```python
from build123d import *

# Parameters (mm, degrees)
SALIENTE_EXTRUIR1_DEPTH = 30
CORTAR_EXTRUIR1_DEPTH   = 5
CROQUIS3_W              = 30
CROQUIS3_H              = 25
CORTAR_EXTRUIR2_DEPTH   = 2
CROQUIS4_R              = 1.35
CROQUIS4_R_2            = 3
CORTAR_EXTRUIR3_DEPTH   = 5
CROQUIS5_W              = 25
CROQUIS5_H              = 25
CORTAR_EXTRUIR4_DEPTH   = 2
REDONDEO1_R             = 15
REDONDEO2_R             = 8
REDONDEO3_R             = 2.7
SALIENTE_EXTRUIR2_DEPTH = 5
REDONDEO4_R             = 5
SALIENTE_EXTRUIR3_START = -3
SALIENTE_EXTRUIR3_DEPTH = 3
SALIENTE_EXTRUIR4_START = -30
SALIENTE_EXTRUIR4_DEPTH = 3
REDONDEO5_R             = 10


with BuildPart() as part:
    # Croquis1 → Saliente-Extruir1 (new body)
    with BuildSketch(Plane.XY):
        with BuildLine():
            Line((0, 0), (0, 5))
            Line((0, 5), (-40, 5))
            ThreePointArc((-40, 5), (-59.427874629, -2.62943546), (-71, -20))
            Line((-71, -20), (-71, -60))
            Line((-71, -60), (-66, -60))
            Line((-66, -60), (-66, -20.535714286))
            ThreePointArc((-66, -20.535714286), (-56.328368106, -6.472823549), (-40.535714286, 0))
            Line((-40.535714286, 0), (0, 0))
        make_face()
    extrude(amount=SALIENTE_EXTRUIR1_DEPTH)

    # Croquis2 → Cortar-Extruir1 (cut)
    with BuildSketch(Plane(origin=(0, 5, 0), x_dir=(1, 0, 0), z_dir=(0, 1, 0))):
        with BuildLine():
            Line((-18.4, -6.93), (-8.4, -6.93))
            ThreePointArc((-8.4, -6.93), (-7.05, -8.28), (-8.4, -9.63))
            Line((-8.4, -9.63), (-28.4, -9.63))
            ThreePointArc((-28.4, -9.63), (-29.75, -8.28), (-28.4, -6.93))
            Line((-28.4, -6.93), (-18.4, -6.93))
        make_face()
        with BuildLine():
            Line((-8.4, -20.37), (-28.4, -20.37))
            ThreePointArc((-28.4, -20.37), (-29.75, -21.72), (-28.4, -23.07))
            Line((-28.4, -23.07), (-18.4, -23.07))
            Line((-18.4, -23.07), (-8.4, -23.07))
            ThreePointArc((-8.4, -23.07), (-7.05, -21.72), (-8.4, -20.37))
        make_face()
    extrude(amount=-CORTAR_EXTRUIR1_DEPTH, mode=Mode.SUBTRACT)

    # Croquis3 → Cortar-Extruir2 (cut)
    with BuildSketch(Plane.XZ):
        with Locations((-18.4, 15)):
            Rectangle(CROQUIS3_W, CROQUIS3_H)
    extrude(amount=-CORTAR_EXTRUIR2_DEPTH, mode=Mode.SUBTRACT)

    # Croquis4 → Cortar-Extruir3 (cut)
    with BuildSketch(Plane.ZY.offset(71)):
        with Locations((22.071067812, -34.528932188)):
            Circle(CROQUIS4_R)
        with Locations((22.071067812, -48.671067812)):
            Circle(CROQUIS4_R)
        with Locations((7.928932188, -48.671067812)):
            Circle(CROQUIS4_R)
        with Locations((7.928932188, -34.528932188)):
            Circle(CROQUIS4_R)
        with Locations((15, -41.6)):
            Circle(CROQUIS4_R_2)
    extrude(amount=-CORTAR_EXTRUIR3_DEPTH, mode=Mode.SUBTRACT)

    # Croquis5 → Cortar-Extruir4 (cut)
    with BuildSketch(Plane.ZY.offset(71)):
        with Locations((15, -41.6)):
            Rectangle(CROQUIS5_W, CROQUIS5_H)
    extrude(amount=-CORTAR_EXTRUIR4_DEPTH, mode=Mode.SUBTRACT)

    # Redondeo1
    # the kernel refuses this fillet: 15 mm, written as the material it adds along each edge
    with BuildSketch(Plane(origin=(-40.535714286, 0, 0), x_dir=(-0.9928040160487852, -0.11975051447657076, 0), z_dir=(0, 0, 1))) as redondeo1_piece_1:
        with BuildLine():
            CenterArc((0.928120739, 14.996773606), REDONDEO1_R, 263.122295715, 8.066092884)
            Line((-0.868136978, 0.104713365), (0, 0))
            ThreePointArc((0, 0), (0.61960892, -0.006425976), (1.23921784, 0))
        make_face()
    extrude(amount=30)
    with BuildSketch(Plane(origin=(-66, -20.535714286, 0), x_dir=(0, -1, 0), z_dir=(0, 0, 1))) as redondeo1_piece_2:
        with BuildLine():
            CenterArc((2.787806423, 15), REDONDEO1_R, 244.497181261, 25.502818739)
            ThreePointArc((-3.670526079, 1.461538444), (-1.859449277, 0.670027601), (0, 0))
            Line((0, 0), (2.787806423, 0))
        make_face()
    extrude(amount=30)
    # the kernel refuses this fillet: 15 mm, written as the material it takes off along each edge
    with BuildSketch(Plane(origin=(-71, -20, -8.10538424), x_dir=(0, -1, 0), z_dir=(0, 0, 1))) as redondeo1_2_piece_1:
        with BuildLine():
            CenterArc((2.445891068, 15), REDONDEO1_R, 248.435113489, 21.564886511)
            ThreePointArc((-3.067429039, 1.049971276), (-1.545944268, 0.48925715), (0, 0))
            Line((0, 0), (2.445891068, 0))
        make_face()
    extrude(amount=46.210768479, mode=Mode.SUBTRACT)
    with BuildSketch(Plane(origin=(-40, 5, -1.977224952), x_dir=(-0.9967130662310812, -0.08101273729628075, 0), z_dir=(0, 0, 1))) as redondeo1_2_piece_2:
        with BuildLine():
            CenterArc((0.620502289, 14.999032237), REDONDEO1_R, 265.35321973, 5.297627307)
            Line((-0.59468877, 0.048336243), (0, 0))
            ThreePointArc((0, 0), (0.39544499, -0.002246038), (0.790889981, 0))
        make_face()
    extrude(amount=33.954449904, mode=Mode.SUBTRACT)

    # Redondeo2
    redondeo2_edges = [part.edges().sort_by_distance(p)[0] for p in [
        (0, 2.5, 0),
        (-68.5, -60, 30),
        (0, 2.5, 30),
        (-68.5, -60, 0),
    ]]
    fillet(redondeo2_edges, radius=REDONDEO2_R)

    # Redondeo3
    redondeo3_edges = [part.edges().sort_by_distance(p)[0] for p in [
        (-70, -29.1, 27.5),
        (-70, -54.1, 27.5),
        (-70, -54.1, 2.5),
        (-70, -29.1, 2.5),
        (-3.4, 1, 27.5),
        (-3.4, 1, 2.5),
        (-33.4, 1, 2.5),
        (-33.4, 1, 27.5),
    ]]
    fillet(redondeo3_edges, radius=REDONDEO3_R)

    # Croquis6 → Saliente-Extruir2 (add)
    with BuildSketch(Plane.XZ):
        with BuildLine():
            Line((0, 22), (0, 8))
            Line((0, 8), (15, 8))
            Line((15, 8), (15, 16))
            Line((15, 16), (13.291287847, 16))
            ThreePointArc((13.291287847, 16), (9.630693606, 12.908349934), (11, 17.5))
            Line((11, 17.5), (15, 17.5))
            Line((15, 17.5), (15, 22))
            Line((15, 22), (0, 22))
        make_face()
    extrude(amount=-SALIENTE_EXTRUIR2_DEPTH)

    # Redondeo4
    # the kernel refuses this fillet: 5 mm, written as the material it adds along each edge
    with BuildSketch(Plane(origin=(0, 0, 22), x_dir=(-0.19611613513818366, 0, 0.9805806756909203), z_dir=(0, 1, 0))) as redondeo4_piece_1:
        with BuildLine():
            CenterArc((4.118438838, 4.902903378), REDONDEO4_R, 191.309932474, 67.380135052)
            Line((-0.784464541, 3.922322703), (0, 0))
            ThreePointArc((0, 0), (1.568929081, 0.155354594), (3.137858162, 0))
        make_face()
    extrude(amount=5)
    with BuildSketch(Plane(origin=(0, 0, 8), x_dir=(-0.19611613513818402, 0, -0.9805806756909201), z_dir=(0, 1, 0))) as redondeo4_piece_2:
        with BuildLine():
            CenterArc((4.118438838, -4.902903378), REDONDEO4_R, 101.309932474, 67.380135052)
            Line((-0.784464541, -3.922322703), (0, 0))
            ThreePointArc((0, 0), (1.568929081, -0.155354594), (3.137858162, 0))
        make_face()
    extrude(amount=5)
    # the kernel refuses this fillet: 5 mm, written as the material it takes off along each edge
    with BuildSketch(Plane(origin=(15, -12.437342964, 22), x_dir=(-1, 0, 0), z_dir=(0, 1, 0))) as redondeo4_2_piece_1:
        with BuildLine():
            CenterArc((4.974937186, -5), REDONDEO4_R, 90, 84.260829523)
            Line((0, -4.5), (0, 0))
            Line((0, 0), (4.974937186, 0))
        make_face()
    extrude(amount=29.874685928, mode=Mode.SUBTRACT)
    with BuildSketch(Plane(origin=(15, -12.5, 8), x_dir=(0, 0, 1), z_dir=(0, 1, 0))) as redondeo4_2_piece_2:
        with BuildLine():
            CenterArc((REDONDEO4_R, -REDONDEO4_R), REDONDEO4_R, 90, 90)
            Line((0, -REDONDEO4_R), (0, 0))
            Line((0, 0), (REDONDEO4_R, 0))
        make_face()
    extrude(amount=30, mode=Mode.SUBTRACT)

    # Croquis9 → Saliente-Extruir3 (add)
    with BuildSketch(Plane.XY.offset(30).offset(SALIENTE_EXTRUIR3_START)):
        with BuildLine():
            Line((-66, -23.323520708), (-39.661284928, 0))
            ThreePointArc((-39.661284928, 0), (-40.716262324, -0.037145236), (-41.766014734, -0.148396974))
            ThreePointArc((-41.766014734, -0.148396974), (-55.25292739, -5.645128922), (-64.538461556, -16.865188206))
            ThreePointArc((-64.538461556, -16.865188206), (-65.630053372, -20.01269931), (-66, -23.323520708))
        make_face()
    extrude(amount=SALIENTE_EXTRUIR3_DEPTH)

    # Croquis9<2> → Saliente-Extruir4 (add)
    with BuildSketch(Plane.XY.offset(30).offset(SALIENTE_EXTRUIR4_START)):
        with BuildLine():
            Line((-66, -23.323520708), (-39.661284928, 0))
            ThreePointArc((-39.661284928, 0), (-40.716262324, -0.037145236), (-41.766014734, -0.148396974))
            ThreePointArc((-41.766014734, -0.148396974), (-55.25292739, -5.645128922), (-64.538461556, -16.865188206))
            ThreePointArc((-64.538461556, -16.865188206), (-65.630053372, -20.01269931), (-66, -23.323520708))
        make_face()
    extrude(amount=SALIENTE_EXTRUIR4_DEPTH)

    # Redondeo5
    redondeo5_edges = [part.edges().sort_by_distance(p)[0] for p in [
        (-39.661284928, 0, 28.5),
        (-66, -23.323520708, 1.5),
        (-66, -23.323520708, 28.5),
        (-39.661284928, 0, 1.5),
    ]]
    fillet(redondeo5_edges, radius=REDONDEO5_R)


solid = part.part
```
Source: CAD feature listing. Evaluate the final solid. Frame: model axes, mm. A direction names the side the tool comes from. Coordinates: 2 decimals unless noted, no trailing zeros. Write each loop counter-clockwise with the first axis right and the second up, starting at its lowest first coordinate (ties: lowest second). Pieces come first, ordered by that corner, then holes. Notation, with made-up numbers: (38.5, 63) -> (85.5, 63) arc R25 cw to (85.5, 83) -> close; hole circle Ø9 at (5, 60.5). An arc over 180 degrees is marked (long way). Return JSON: item names as keys, results as strings. Group by question number.
1) Set-up query: faces 1 (the face through (-33.4, 1, 15)), 2 (the face through (-69.99, -53.33, 26.69)), 3 (the face through (7, 2, 22)), 4 (the face through (-55, -10, 27)). Return all of +Z, -Z, +X, -X, +Y, -Y with unobstructed straight access to the full face (end or side cutting, diameter ignored); none if empty.
2) Mould query, pull axis X, two halves, no side actions, for faces 5 (the face through (-52.705, -11.551, 1.479)), 6 (the face through (-29.75, 3.52, 8.31)), 7 (the face through (13, 2, 17.5)). Classes: +X half, -X half, draft (parallel to the pull), parting line (faces both ways), or undercut.
3) Section query A-A, the plane z = 15. Return loops of the section in (x, y), plus the area to 3 significant figures.
4) Ray query, line 1 along Y through (x, z) = (-13, 14.5); line 2 along X through (y, z) = (-46, 15); line 3 along Y through (x, z) = (-38, 26.25). Return the intervals inside material, ascending.
5) Section query B-B, the plane x = -18.5. Return loops of the section in (y, z).
6) Section query C-C, the plane y = -8. Return loops of the section in (x, z), plus the area to 3 significant figures.
7) Section query D-D, the plane z = 26. Return loops of the section in (x, y).
8) Contact query for flat-ended pins moving along their axis: P1, Ø3, axis at x = 13.5, y = 2, coming from the -Z side; P2, Ø10, axis at x = -61.5, z = 10.5, coming from the +Y side; P3, Ø7.5, axis at y = -40, z = 12, coming from the -X side. Output: stop coordinate, or through.
From the geometry:
{
 "1": {"face 1": "-Y", "face 2": "-X", "face 3": "+Z, +X, +Y, -Y", "face 4": "+X, -Y"},
 "2": {"face 5": "+X half", "face 6": "undercut", "face 7": "draft"},
 "3": {"outline": "(-71, -60) -> (-66, -60) -> (-66, -44.6) -> (-69, -44.6) -> (-69, -54.1) -> (-71, -54.1) -> close; (-71, -29.1) -> (-69, -29.1) -> (-69, -38.6) -> (-66, -38.6) -> (-66, -23.32) arc R15 cw to (-64.54, -16.87) arc R29.88 cw to (-41.77, -0.15) arc R15 cw to (-39.66, 0) -> (-33.4, 0) -> (-33.4, 2) -> (-3.4, 2) -> (-3.4, 0) -> (8.5, 0) -> (8.5, 5) -> (-39.4, 5) arc R15 ccw to (-40.79, 4.94) arc R34.81 ccw to (-69.95, -16.93) arc R15 ccw to (-71, -22.45) -> close; (13.5, 0) -> (15, 0) -> (15, 5) -> (13.5, 5) -> close", "area": "512 mm²"},
 "4": {"line 1": "2 to 5", "line 2": "-69 to -66", "line 3": "0 to 5"},
 "5": {"outline": "(0, 0) -> (5, 0) -> (5, 6.93) -> (2, 6.93) -> (2, 2.5) -> (0, 2.5) -> close; (0, 27.5) -> (2, 27.5) -> (2, 23.07) -> (5, 23.07) -> (5, 30) -> (0, 30) -> close; (2, 9.63) -> (5, 9.63) -> (5, 20.37) -> (2, 20.37) -> close"},
 "6": {"outline": "(-64.77, 0) -> (-48.7, 0) -> (-48.7, 3) -> (-58.08, 3) -> (-58.08, 27) -> (-48.7, 27) -> (-48.7, 30) -> (-64.77, 30) -> close", "area": "257 mm²"},
 "7": {"outline": "(-71, -58.93) -> (-66, -58.93) -> (-66, -23.32) arc R15 cw to (-64.54, -16.87) arc R29.88 cw to (-41.77, -0.15) arc R15 cw to (-39.66, 0) -> (-33.12, 0) -> (-33.12, 2) -> (-3.68, 2) -> (-3.68, 0) -> (-1.07, 0) -> (-1.07, 5) -> (-39.4, 5) arc R15 ccw to (-40.79, 4.94) arc R34.81 ccw to (-69.95, -16.93) arc R15 ccw to (-71, -22.45) -> (-71, -29.38) -> (-69, -29.38) -> (-69, -53.82) -> (-71, -53.82) -> close"},
 "8": {"P1": "z = 8.42", "P2": "y = -0.51", "P3": "x = -69"}
}
